Here's how the part is built. I have some questions about the finished solid (model axes, mm). A direction names the side the tool comes from. Give positions to 0.01 mm unless a question says otherwise; leave off trailing zeros. Order: outer loops, then holes, each group sorted by start corner. A loop starts at its lowest first (then second) coordinate and runs counter-clockwise, first axis right, second up. Notation, with made-up numbers: M 65.5,-10.75 L 86.5,-10.75 A18 cw 86.5,-4.75 Z; hole C 46,7 d2. An arc over 180 degrees is marked long. Use CSV: the item, a comma, the result in double quotes. Start each with the question number.
```python
from build123d import *

# Parameters (mm, degrees)
SKETCH2_W           = 105.7275
SKETCH2_H           = 105.7275
BOSS_EXTRUDE1_DEPTH = 4.7625
BOSS_EXTRUDE2_DEPTH = 31.75
SKETCH6_R           = 2.099999991
CUT_EXTRUDE1_DEPTH  = 154.914817899
FILLET1_R           = 6.35
SKETCH7_W           = 62.865
SKETCH7_H           = 62.865
CUT_EXTRUDE2_DEPTH  = 153.855065381


with BuildPart() as part:
    # Sketch2 → Boss-Extrude1 (new body)
    with BuildSketch(Plane(origin=(0, 0, 0), x_dir=(1, 0, 0), z_dir=(0, 1, 0))):
        with Locations((52.86375, 52.86375)):
            Rectangle(SKETCH2_W, SKETCH2_H)
    extrude(amount=BOSS_EXTRUDE1_DEPTH)

    # Sketch5 → Boss-Extrude2 (add)
    with BuildSketch(Plane(origin=(0, 0, 0), x_dir=(1, 0, 0), z_dir=(0, 1, 0))):
        Polygon((105.7275, 9.525), (105.7275, 105.7275), (9.525, 105.7275), (9.525, 100.965), (100.965, 100.965), (100.965, 9.525), align=None)
    extrude(amount=-BOSS_EXTRUDE2_DEPTH)

    # Sketch6 → Cut-Extrude1 (cut, through all)
    with BuildSketch(Plane(origin=(0, 4.7625, 0), x_dir=(1, 0, 0), z_dir=(0, 1, 0))):
        with Locations(Location((3.175, 3.175, 0), (0, 0, 270))):
            Circle(SKETCH6_R)
        with Locations(Location((60.325, 4.7625, 0), (0, 0, 270))):
            Circle(SKETCH6_R)
        with Locations(Location((4.7625, 60.325, 0), (0, 0, 270))):
            Circle(SKETCH6_R)
    extrude(amount=-CUT_EXTRUDE1_DEPTH, mode=Mode.SUBTRACT)

    # Fillet1
    # the kernel refuses this fillet: 6.35 mm, written as the material it takes off along each edge
    with BuildSketch(Plane(origin=(9.525, -31.75, -100.965), x_dir=(0, 0, -1), z_dir=(1, 0, 0)), Plane(origin=(100.965, -31.75, -100.965), x_dir=(1, 0, 0), z_dir=(0, 0, 1))) as fillet1_piece_1:
        with BuildLine():
            CenterArc((6.35, 6.148361062), FILLET1_R, 180, 75.522487814)
            Line((0, 6.148361062), (-0.127, 6.148361062))
            Line((-0.127, 6.148361062), (-0.127, 0))
            Line((-0.127, 0), (0, -0.127))
            ThreePointArc((0, -0.127), (2.38125, -0.127), (4.73075, -0.122967221))
            Line((4.73075, -0.122967221), (4.7625, 0))
        make_face()
    extrude(amount=91.44, mode=Mode.SUBTRACT)
    with BuildSketch(Plane(origin=(9.525, -31.75, -100.965), x_dir=(0, 0, -1), z_dir=(1, 0, 0))) as fillet1_piece_2a_section:
        with BuildLine():
            CenterArc((6.35, 6.148361062), FILLET1_R, 180, 75.522487814)
            Line((0, 6.148361062), (-0.127, 6.148361062))
            Line((-0.127, 6.148361062), (-0.127, 0))
            Line((-0.127, 0), (0, -0.127))
            ThreePointArc((0, -0.127), (2.38125, -0.127), (4.73075, -0.122967221))
            Line((4.73075, -0.122967221), (4.7625, 0))
        make_face()
    fillet1_piece_2a = extrude(amount=106.810902655, mode=Mode.PRIVATE)
    fillet1_piece_2a = split(fillet1_piece_2a, bisect_by=Plane(origin=(100.965, -30.30128496, -102.168907648), z_dir=(1, 0, 0)), keep=Keep.TOP, mode=Mode.PRIVATE)
    with BuildSketch(Plane(origin=(100.965, -31.75, -116.335902655), x_dir=(1, 0, 0), z_dir=(0, 0, 1))) as fillet1_piece_2b_section:
        with BuildLine():
            CenterArc((6.35, 6.148361062), FILLET1_R, 180, 75.522487814)
            Line((0, 6.148361062), (-0.127, 6.148361062))
            Line((-0.127, 6.148361062), (-0.127, 0))
            Line((-0.127, 0), (0, -0.127))
            ThreePointArc((0, -0.127), (2.38125, -0.127), (4.73075, -0.122967221))
            Line((4.73075, -0.122967221), (4.7625, 0))
        make_face()
    fillet1_piece_2b = extrude(amount=106.810902655, mode=Mode.PRIVATE)
    fillet1_piece_2b = split(fillet1_piece_2b, bisect_by=Plane(origin=(102.168907648, -30.30128496, -100.965), z_dir=(0, 0, -1)), keep=Keep.TOP, mode=Mode.PRIVATE)
    fillet1_piece_2 = fillet1_piece_2a & fillet1_piece_2b
    add(fillet1_piece_2, mode=Mode.SUBTRACT)

    # Sketch7 → Cut-Extrude2 (cut, through all)
    with BuildSketch(Plane.XZ):
        with Locations((50.4825, -50.4825)):
            Rectangle(SKETCH7_W, SKETCH7_H)
    extrude(amount=-CUT_EXTRUDE2_DEPTH, mode=Mode.SUBTRACT)


solid = part.part
```
Q1. Imagine slicing it at C-C, the plane y = -15. Please give me the cut outline in (x, z) (1 decimal).
Q2. I need wall thicknesses on line 1 (Y direction, x = 8, z = -46.5); line 2 (X direction, y = -18.5, z = -39) (1 decimal); line 3 (Z direction, x = 71, y = -18) (1 decimal). Which ranges of each line are inside material? Lowest first, please. Write a range as [from, to].
Q3. We'd pull the mould along X, two halves only. Please class faces 1 (the face through (54, -13, -105.728)), 2 (the face through (100.965, -13, -56)), 3 (the face through (3.267, 2.415, -5.273)), 4 (the face through (50, 2, -81.915)): pulls with the +X half, pulls with the -X half, needs draft (parallel to the pull), parting line crosses it, or undercut.
Q4. For P1, Ø5, axis at y = -22, z = -103, coming from the -X side (3 decimals); P2, Ø6.5, axis at x = 3.175, z = -3.175, coming from the -Y side; P3, Ø13, axis at y = -18, z = -33, coming from the -X side (3 decimals), each with a flat end and sliding along its axis, tell me the tip position at first contact or that it passes through.
Q5. For faces 5 (the face through (103, -16, -9.525)), 6 (the face through (9.525, -16, -103)), 7 (the face through (50, 2, -19.05)), 8 (the face through (56.953, -29.444, -102.259)), which set-ups out of +Z, -Z, +X, -X, +Y, -Y let a thin tool reach every point of the face, with its end or its side?
Reply:
1,outline,"M 9.5,-105.7 L 105.7,-105.7 L 105.7,-9.5 L 101,-9.5 L 101,-101 L 9.5,-101 Z"
2,line 1,"y = [0, 4.76]"
2,line 2,"x = [101, 105.7]"
2,line 3,"z = [-105.7, -101]"
3,face 1,"needs draft"
3,face 2,"pulls with the -X half"
3,face 3,"undercut"
3,face 4,"undercut"
4,P1,"stops at x = 9.525"
4,P2,"stops at y = 0"
4,P3,"stops at x = 100.965"
5,face 5,"+Z, +X, -X, -Y"
5,face 6,"+Z, -Z, -X, -Y"
5,face 7,"+Y, -Y"
5,face 8,"+Z, -X, -Y"
